Design review of the part built by this model. Coordinates are the model's own, in mm. A direction names the side the tool comes from. Round coordinates to 2 decimals unless told otherwise and drop trailing zeros. Loops run counter-clockwise (first coordinate to the right, second up) from the corner with the lowest first, then second, coordinate; pieces in that order, holes last. Notation, with made-up numbers: (14, -17) - (59, -17) arc R9 ccw to (59, -4) - close; hole circle Ø10 at (26.25, 16.5). An arc over 180 degrees is marked (long way). Use one line per item in the form item = value. Start each with the question number.
(1) We need section C-C, the plane x = 24. Write out the cut boundary in (y, z).
(2) For pin 1 (12.5 mm diameter, centred on x = 68, y = 12.5, fed in from +Z); pin 2 (5 mm diameter, centred on x = 50.5, z = 51.5, fed in from -Y); pin 3 (10 mm diameter, centred on y = -25.5, z = 74, fed in from +X); pin 4 (5 mm diameter, centred on y = 15, z = 46, fed in from -X), all flat-tipped, find the tip position at first contact; note any pin that passes through.
(3) Wall thickness on probe 1 along X at (y, z) = (2.5, 35); probe 2 along X at (y, z) = (21, 87): over which ranges is each line inside the solid? List them lowest first. Write a range as [from, to].
(4) The part is to be moulded in two halves that separate along X. For faces 1 (the flat face through (50.8, 13, 38)), 2 (the flat face through (39, 25.4, 16)), 3 (the flat face through (0, 5, 61)), say which applies: released by +X, released by -X, zero draft, split by the parting line, or undercut.
(5) Machinability: for faces 4 (the flat face through (25.4, 5, 71)), 5 (the flat face through (89, 13, 25.4)), 6 (the flat face through (13, -25, 76.2)), which of the approach directions +Z, -Z, +X, -X, +Y, -Y give a long, thin tool a straight path to every point of the face, cutting with its end or side? Answer none if there is none.
(6) We need section D-D, the plane z = 63. Write out the cut boundary in (x, y).
(7) We need section A-A, the plane z = 29.5. Write out the cut boundary in (x, y), then the cut area to 3 significant figures.
(8) We need section B-B, the plane y = 16.5. Write out the cut boundary in (x, z).
from build123d import *

# Parameters (mm, degrees)
F0_W     = 25.4
F0_H     = 25.4
F1_DEPTH = 25.4
F2_DEPTH = 50.8
F3_DEPTH = 101.6
F4_W     = 25.4
F4_H     = 25.4
F5_DEPTH = 50.8


with BuildPart() as f1:
    # F0 (on Top) → F1 (new body)
    with BuildSketch(Plane.XY):
        with Locations((38.1, 12.7)):
            Rectangle(F0_W, F0_H)
        with Locations((88.9, 12.7)):
            Rectangle(F0_W, F0_H)
    extrude(amount=F1_DEPTH)

    # F0 (on Top) → F2 (join)
    with BuildSketch(Plane.XY):
        with Locations((63.5, 12.7)):
            Rectangle(F0_W, F0_H)
    extrude(amount=F2_DEPTH)

    # F0 (on Top) → F3 (join)
    with BuildSketch(Plane.XY):
        with Locations((12.7, 12.7)):
            Rectangle(F0_W, F0_H)
    extrude(amount=F3_DEPTH)

    # F4 (on face) → F5 (join)
    with BuildSketch(Plane.XZ):
        with Locations((12.7, 88.9)):
            Rectangle(F4_W, F4_H)
    extrude(amount=F5_DEPTH)


solid = f1.part
Data:
q1.outline = (-50.8, 76.2) - (0, 76.2) - (0, 0) - (25.4, 0) - (25.4, 101.6) - (-50.8, 101.6) - close
q2.pin_1 = 50.8
q2.pin_2 = 0
q2.pin_3 = 25.4
q2.pin_4 = 0
q3.probe_1 = [0, 25.4], [50.8, 76.2]
q3.probe_2 = [0, 25.4]
q4.face_1 = undercut
q4.face_2 = zero draft
q4.face_3 = released by -X
q5.face_4 = +Z, +Y, -Y
q5.face_5 = +Z, +X, +Y, -Y
q5.face_6 = -Z, +X, -X, -Y
q6.outline = (0, 0) - (25.4, 0) - (25.4, 25.4) - (0, 25.4) - close
q7.outline = (0, 0) - (25.4, 0) - (25.4, 25.4) - (0, 25.4) - close; (50.8, 0) - (76.2, 0) - (76.2, 25.4) - (50.8, 25.4) - close
q7.area = 1,290 mm^2
q8.outline = (0, 0) - (101.6, 0) - (101.6, 25.4) - (76.2, 25.4) - (76.2, 50.8) - (50.8, 50.8) - (50.8, 25.4) - (25.4, 25.4) - (25.4, 101.6) - (0, 101.6) - close
